from build123d import *

# Parameters (mm, degrees)
SKETCH2_W           = 19
SKETCH2_H           = 20
BOSS_EXTRUDE1_DEPTH = 12
CUT_EXTRUDE1_DEPTH  = 25.596747752
FILLET1_R           = 5
FILLET2_R           = 0.3
SKETCH4_R           = 2.55
CUT_EXTRUDE2_DEPTH  = 2
SKETCH5_R           = 2.9
CUT_EXTRUDE3_DEPTH  = 6
SKETCH6_W           = 19
SKETCH6_H           = 10
BOSS_EXTRUDE2_DEPTH = 10
SKETCH7_R           = 2.15
CUT_EXTRUDE4_DEPTH  = 25.596747919
FILLET3_R           = 5


# Some blends are built 0.0001 mm under size
with BuildPart() as part:
    # Sketch2 → Boss-Extrude1 (new body)
    with BuildSketch(Plane(origin=(0, 0, 0), x_dir=(1, 0, 0), z_dir=(0, 1, 0))):
        Rectangle(SKETCH2_W, SKETCH2_H)
    extrude(amount=BOSS_EXTRUDE1_DEPTH)

    # Sketch3 → Cut-Extrude1 (cut, through all)
    with BuildSketch(Plane(origin=(9.5, 0, 0), x_dir=(0, 0, -1), z_dir=(1, 0, 0))):
        Polygon((-3.8, 12), (3.8, 12), (5.25, 8.890464965), (-5.25, 8.890464965), align=None)
    extrude(amount=-CUT_EXTRUDE1_DEPTH, mode=Mode.SUBTRACT)

    # Fillet1
    # the kernel refuses this fillet: 5 mm, written as the material it takes off along each edge
    with BuildSketch(Plane(origin=(-9.5, -12.5, -10), x_dir=(1, 0, 0), z_dir=(0, 1, 0)), Plane(origin=(-9.5, -12.5, 10), x_dir=(0, 0, -1), z_dir=(0, 1, 0))) as fillet1_piece_1:
        with BuildLine():
            CenterArc((FILLET1_R, -FILLET1_R), FILLET1_R, 90, 90)
            Line((0, -FILLET1_R), (0, 0))
            Line((0, 0), (FILLET1_R, 0))
        make_face()
    extrude(amount=37, mode=Mode.SUBTRACT)
    with BuildSketch(Plane(origin=(9.5, -12.5, -10), x_dir=(-1, 0, 0), z_dir=(0, 1, 0)), Plane(origin=(9.5, -12.5, 10), x_dir=(0, 0, -1), z_dir=(0, 1, 0))) as fillet1_piece_2:
        with BuildLine():
            CenterArc((FILLET1_R, FILLET1_R), FILLET1_R, 180, 90)
            Line((0, FILLET1_R), (0, 0))
            Line((0, 0), (FILLET1_R, 0))
        make_face()
    extrude(amount=37, mode=Mode.SUBTRACT)

    # Fillet2
    fillet2_edges = [part.edges().sort_by_distance(p)[0] for p in [
        (0, 12, 3.8),
        (0, 12, -3.8),
        (0, 8.890464965, -5.25),
        (0, 8.890464965, 5.25),
    ]]
    fillet(fillet2_edges, radius=FILLET2_R)

    # Sketch4 → Cut-Extrude2 (cut)
    with BuildSketch(Plane(origin=(0, 8.890464965, 0), x_dir=(1, 0, 0), z_dir=(0, 1, 0))):
        with Locations(Location((0, 0, 0), (0, 0, 270))):
            Circle(SKETCH4_R)
    extrude(amount=-CUT_EXTRUDE2_DEPTH, mode=Mode.SUBTRACT)

    # Sketch5 → Cut-Extrude3 (cut)
    with BuildSketch(Plane(origin=(0, 6.890464965, 0), x_dir=(1, 0, 0), z_dir=(0, 1, 0))):
        with Locations(Location((0, 0, 0), (0, 0, 270))):
            Circle(SKETCH5_R)
    extrude(amount=-CUT_EXTRUDE3_DEPTH, mode=Mode.SUBTRACT)

    # Sketch6 → Boss-Extrude2 (add)
    with BuildSketch(Plane.XZ):
        Rectangle(SKETCH6_W, SKETCH6_H)
    extrude(amount=BOSS_EXTRUDE2_DEPTH)

    # Sketch7 → Cut-Extrude4 (cut, through all)
    with BuildSketch(Plane(origin=(9.5, 0, 0), x_dir=(0, 0, -1), z_dir=(1, 0, 0))):
        with Locations((0, -5)):
            Circle(SKETCH7_R)
    extrude(amount=-CUT_EXTRUDE4_DEPTH, mode=Mode.SUBTRACT)

    # Fillet3
    fillet3_edges = [part.edges().sort_by_distance(p)[0] for p in [
        (0, -10, -5),
        (0, -10, 5),
    ]]
    fillet(fillet3_edges, radius=FILLET3_R - 0.0001)  # a hair under: the kernel refuses the full size


solid = part.part
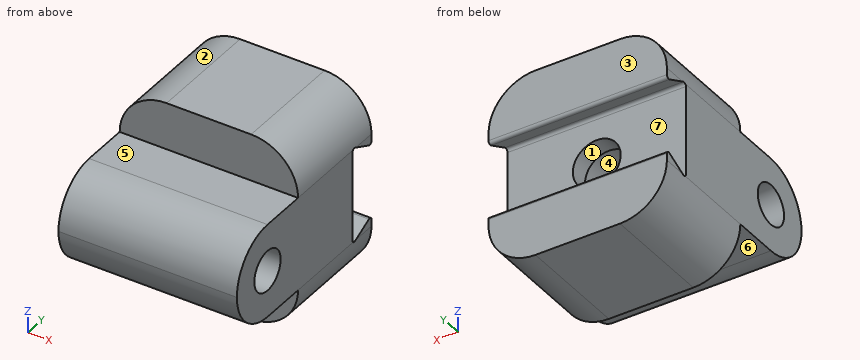
Could you check a few things on this model? Use its own coordinates, in mm. Face numbers are marked on the shaded views. A direction names the side the tool comes from. Round coordinates to 2 decimals unless told otherwise and drop trailing zeros. Write each loop counter-clockwise with the first axis right and the second up, starting at its lowest first coordinate (ties: lowest second). Pieces come first, ordered by that corner, then holes. Notation, with made-up numbers: (76.25, 33) -> (119.25, 33) arc R12 ccw to (119.25, 48) -> close; hole circle Ø1 at (37, 65.25). An arc over 180 degrees is marked (long way). Use a Markdown table: item, result.
1. Please list where these lines run through material, in increasing order: probe 1 along X at (y, z) = (3.4, 0); probe 2 along Y at (x, z) = (8.75, -7.5); probe 3 along Z at (x, y) = (6.75, 9.5).
Answer key:
| item | result |
|---|---|
| probe 1 | x = -9.5 to -2.9, 2.9 to 9.5 |
| probe 2 | y = 0 to 12 |
| probe 3 | z = -9.47 to -4.97, 4.97 to 9.47 |
2. If we section it at C-C (z = 0.5): List the corners of the cut face in (x, y) for me, then the cut area to 3 significant figures.
Answer key:
| item | result |
|---|---|
| outline | (-9.5, -9.97) -> (9.5, -9.97) -> (9.5, -7.09) -> (-9.5, -7.09) -> close; (-9.5, -2.91) -> (9.5, -2.91) -> (9.5, 8.89) -> (2.5, 8.89) -> (2.5, 6.89) -> (2.86, 6.89) -> (2.86, 0.89) -> (-2.86, 0.89) -> (-2.86, 6.89) -> (-2.5, 6.89) -> (-2.5, 8.89) -> (-9.5, 8.89) -> close |
| area | 235 mm^2 |
3. Which directions (+Z, -Z, +X, -X, +Y, -Y) give clear straight access to the entire face, cutting with the end or side of a thin tool? Please do the marked faces 5, 6 and 7.
Answer key:
| item | result |
|---|---|
| face 5 | +Z, +X, -X, -Y |
| face 6 | -Z, +X, -X, -Y |
| face 7 | +X, -X |
4. If we section it at D-D (y = -6.5): List the corners of the cut face in (x, z) for me, then the cut area to 3 significant figures.
Answer key:
| item | result |
|---|---|
| outline | (-9.5, -4.77) -> (9.5, -4.77) -> (9.5, -1.54) -> (-9.5, -1.54) -> close; (-9.5, 1.54) -> (9.5, 1.54) -> (9.5, 4.77) -> (-9.5, 4.77) -> close |
| area | 123 mm^2 |
5. If we section it at B-B (y = 5.5): List the corners of the cut face in (x, z) for me.
Answer key:
| item | result |
|---|---|
| outline | (-9.5, -5) arc R5 ccw to (-4.5, -10) -> (4.5, -10) arc R5 ccw to (9.5, -5) -> (9.5, 5) arc R5 ccw to (4.5, 10) -> (-4.5, 10) arc R5 ccw to (-9.5, 5) -> close; hole circle Ø5.8 at (0, 0) |
6. For pin 1 Ø4.5 at (x, z) = (-1, 1) entering from +Y; pin 2 Ø4 at (y, z) = (-2, -6.5) entering from +X; pin 3 Ø1.5 at (x, y) = (-2.5, -2.5) entering from -Z; pin 4 Ø2.5 at (x, z) = (1, 7) entering from -Y, each with a flat end and sliding along its axis, tell me the tip position at first contact or that it passes through.
Answer key:
| item | result |
|---|---|
| pin 1 | stops at y = 8.89 |
| pin 2 | stops at x = 9.5 |
| pin 3 | stops at z = -5 |
| pin 4 | stops at y = 0 |
7. We'd pull the mould along Z, two halves only. Please class the marked faces 1, 2, 3 and 4: +Z half, -Z half, draft (parallel to the pull), parting line (faces both ways), or undercut.
Answer key:
| item | result |
|---|---|
| face 1 | undercut |
| face 2 | +Z half |
| face 3 | draft |
| face 4 | undercut |
